For this review, take the finished solid that the model builds, in its own axes (mm). A direction names the side the tool comes from. Give positions to 0.01 mm unless a question says otherwise; leave off trailing zeros. Loops run counter-clockwise (first coordinate to the right, second up) from the corner with the lowest first, then second, coordinate; pieces in that order, holes last. Notation, with made-up numbers: (-15.75, -15) - (39.25, -15) arc R28 ccw to (39.25, 8) - close; hole circle Ø8 at (-33.5, 44.5). An arc over 180 degrees is marked (long way). Answer in a Markdown table with one row per item.
Solid Edge part; units mm, degrees
sketch "Sketch1" plane through (0, 0, 0) normal (0, -1, 0) x (1, 0, 0)
  line L0 (-40, 60) -> (40, 60)
  line L1 (40, 60) -> (70, 70)
  line L2 (70, 70) -> (100, 70)
  arc A0 (100, 70) -> (100, -80) centre (-30.625, -5) cw
  line L3 (-100, -80) -> (100, -80)
  arc A1 (-100, 70) -> (-100, -80) centre (30.625, -5) ccw
  line L4 (-70, 70) -> (-100, 70)
  line L5 (-40, 60) -> (-70, 70)
  dimension "D1" = 70
  dimension "D2" = 70
  dimension "D3" = 70
extrude "Protrusion1" add sketch "Sketch1" along normal blind 5
fillet "Round_1" radius 30 8 edges at (100, -2.5, -80) (-100, -2.5, -80) (-100, -2.5, 70) (-70, -2.5, 70) (-40, -2.5, 60) (40, -2.5, 60) (70, -2.5, 70) (100, -2.5, 70)
sketch "Sketch2" plane through (0, -5, -2.5) normal (0, -1, 0) x (1, 0, 0)
  circle A0 centre (0, 2.5) radius 27.5
extrude "ExtrudedCutout_1" cut sketch "Sketch2" against normal blind 45.5 and the other way blind 29.5
hole "Hole_1" at (0, -5, 35) direction (0, 1, 0) diameter 6 end up to next
pattern_circular "Pattern1" count 6 over 360 about axis through (0, -5, 0) along (0, 1, 0) of "Hole_1"
sketch "Sketch3" plane through (0, -5, -5) normal (0, -1, 0) x (1, 0, 0)
  arc A0 (-72.1237, 40.2166) -> (-55.3222, 36.6862) centre (-68.3481, 16.44) cw
  arc A1 (-55.3222, 36.6862) -> (-51.18, 25.3196) centre (-60.7329, 28.2764) cw
  arc A2 (-51.18, 25.3196) -> (-50.4231, -27.6469) centre (30.625, 0) ccw
  arc A3 (-53.6794, -39.3255) -> (-50.4231, -27.6469) centre (-59.7121, -31.3501) ccw
  arc A4 (-53.6794, -39.3255) -> (-74.0366, -41.5749) centre (-65.7448, -23.3747) cw
  arc A5 (-74.0366, -41.5749) -> (-79.4063, -35.5491) centre (-69.8907, -32.4748) cw
  arc A6 (-79.4063, -35.5491) -> (-80.134, 33.2126) centre (30.625, 0) cw
  arc A7 (-80.134, 33.2126) -> (-72.1237, 40.2166) centre (-70.5554, 30.3403) cw
extrude "ExtrudedCutout_2" cut sketch "Sketch3" against normal blind 23.5 and the other way blind 37.5
mirror "Mirror1" about plane through (0, 0, 0) normal (1, 0, 0) of "ExtrudedCutout_2"
properties material "Epoxy, cast rigid"
1. We need section C-C, the plane y = -3.1. Count the separate pieces of the cut face and the enclosed holes in it, and give its area (3 significant figures).
Values:
| item | result |
|---|---|
| separate pieces | 1 |
| enclosed holes | 9 |
| area | 25,300 mm^2 |
2. Wall thickness on line 1 (Z direction, x = 0, y = -2.65); line 2 (X direction, y = -4.8, z = -12); line 3 (X direction, y = -1.15, z = -37): over which ranges is each line inside the solid? List them lowest first. Write a range as [from, to].
Values:
| item | result |
|---|---|
| line 1 | z = [-80, -38], [-32, -27.5], [27.5, 32], [38, 60] |
| line 2 | x = [-119.84, -84.79], [-54.72, -24.74], [24.74, 54.72], [84.79, 119.84] |
| line 3 | x = [-116.56, -80.49], [-49.73, -2.24], [2.24, 49.73], [80.49, 116.56] |
3. We need section B-B, the plane z = 23.5. Give the boundary of the cut face in (x, y).
Values:
| item | result |
|---|---|
| outline | (-117.28, -5) - (-81.44, -5) - (-81.44, 0) - (-117.28, 0) - close; (-50.74, -5) - (-14.28, -5) - (-14.28, 0) - (-50.74, 0) - close; (14.28, -5) - (50.74, -5) - (50.74, 0) - (14.28, 0) - close; (81.44, -5) - (117.28, -5) - (117.28, 0) - (81.44, 0) - close |
4. Clearance check with flat-ended pins moving along their axes: pin 1 (5 mm diameter, centred on x = 61.5, z = -46, fed in from +Y); pin 2 (3.5 mm diameter, centred on x = 30.31, z = -17.5, fed in from +Y); pin 3 (3 mm diameter, centred on y = -3.5, z = -49.5, fed in from +X); pin 4 (2 mm diameter, centred on y = -3.5, z = -58.5, fed in from +X). State where each tip first meets the part, or that it passes through.
Values:
| item | result |
|---|---|
| pin 1 | stops at y = 0 |
| pin 2 | passes through |
| pin 3 | stops at x = 113.73 |
| pin 4 | stops at x = 110.55 |
5. We need section A-A, the plane x = 0. Give the boundary of the cut face in (y, z), and give its area (3 significant figures).
Values:
| item | result |
|---|---|
| outline | (-5, -80) - (0, -80) - (0, -38) - (-5, -38) - close; (-5, -32) - (0, -32) - (0, -27.5) - (-5, -27.5) - close; (-5, 27.5) - (0, 27.5) - (0, 32) - (-5, 32) - close; (-5, 38) - (0, 38) - (0, 60) - (-5, 60) - close |
| area | 365 mm^2 |
6. Mouldability with a two-part tool opening along Z and no side actions: class faces 1 (the face through (-63.7, -2.54, -48.27)), 2 (the face through (77.197, -2.535, 32.817)), 3 (the face through (28, -5, -6)), 4 (the face through (-78, -2, 70)) as released by +Z, released by -Z, zero draft, split by the parting line, or undercut.
Values:
| item | result |
|---|---|
| face 1 | undercut |
| face 2 | undercut |
| face 3 | zero draft |
| face 4 | released by +Z |
7. We need section D-D, the plane x = 91. Give the boundary of the cut face in (y, z), and give its area (3 significant figures).
Values:
| item | result |
|---|---|
| outline | (-5, -78.39) - (0, -78.39) - (0, 68.39) - (-5, 68.39) - close |
| area | 734 mm^2 |
8. For faces 5 (the face through (39.87, -2.535, 60.377)), 6 (the face through (-77.4, -2.54, -44.08)), 7 (the face through (-98.29, -2.54, -74.72)), list the 3-axis set-ups (+Z, -Z, +X, -X, +Y, -Y) from which the entire face can be reached by the end or side of a thin tool; tool diameter is ignored.
Values:
| item | result |
|---|---|
| face 5 | +Z, +Y, -Y |
| face 6 | +Y, -Y |
| face 7 | -Z, -X, +Y, -Y |
